Print and shaded views of the part. All mm, measured from the part's lowest x, y and z. A direction names the side the tool comes from. Coordinates: 2 decimals unless noted, no trailing zeros. Loops run counter-clockwise (first coordinate to the right, second up) from the corner with the lowest first, then second, coordinate; pieces in that order, holes last. Notation, with made-up numbers: M 56,80.25 L 100,80.25 A12 cw 100,101.25 Z; hole C 16.5,63 d3. An arc over 180 degrees is marked long. One line per question, with ' | ' between items. Start each with the question number.
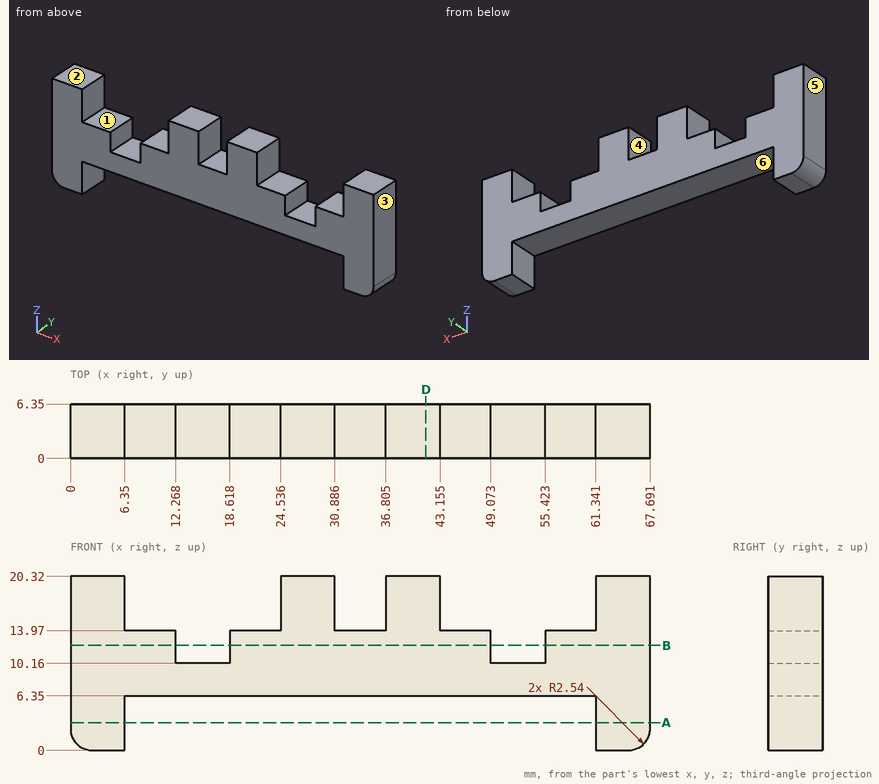
(1) Drill centre lines: line 1 (X direction, y = 0.75, z = 12.25); line 2 (X direction, y = 4.75, z = 6); line 3 (Z direction, x = 40, y = 5.5). Where is each one in solid material? Low to high. Write a range as [from, to].
(2) Band-saw the part on A-A on z = 3.25. Write the cut outline in (x, y).
(3) Pin check, flat tips, straight feed: P1, Ø5, axis at x = 20, z = 18, coming from the +Y side; P2, Ø2, axis at x = 40.5, y = 2.5, coming from the -Z side; P3, Ø3, axis at x = 59.5, y = 3.5, coming from the +Z side. Stop position of each tip, or through.
(4) Two-plate mould, pull along X, no slides. Class the marked faces 1, 2 and 3: pulls with the +X half, pulls with the -X half, needs draft (parallel to the pull), parting line crosses it, or undercut.
(5) Band-saw the part on D-D on x = 41.5. Write the cut outline in (y, z).
(6) 3-axis set-ups, long thin cutter, end or side, ignore diameter. For the marked faces 4, 5 and 6: which of +Z, -Z, +X, -X, +Y, -Y reach the whole face in a straight line?
(7) Band-saw the part on B-B on z = 12.25. Write the cut outline in (x, y), then the cut area to 3 significant figures.
Computed values:
1) line 1: [0, 12.27], [18.62, 49.07], [55.42, 67.69] | line 2: [0, 6.35], [61.34, 67.69] | line 3: [6.35, 20.32]
2) outline: M 0,0 L 6.35,0 L 6.35,6.35 L 0,6.35 Z; M 61.34,0 L 67.69,0 L 67.69,6.35 L 61.34,6.35 Z
3) P1: through | P2: z = 6.35 | P3: z = 13.97
4) face 1: undercut | face 2: needs draft | face 3: pulls with the +X half
5) outline: M 0,6.35 L 6.35,6.35 L 6.35,20.32 L 0,20.32 Z
6) face 4: +Z, +Y, -Y | face 5: +Z, -Z, -X, +Y, -Y | face 6: -Z, +Y, -Y
7) outline: M 0,0 L 12.27,0 L 12.27,6.35 L 0,6.35 Z; M 18.62,0 L 49.07,0 L 49.07,6.35 L 18.62,6.35 Z; M 55.42,0 L 67.69,0 L 67.69,6.35 L 55.42,6.35 Z | area: 349 mm^2
